For this review, take the finished solid that the model builds, in its own axes (mm). Face numbers are marked on the shaded views. Coordinates: 2 decimals unless noted, no trailing zeros. Loops run counter-clockwise (first coordinate to the right, second up) from the corner with the lowest first, then second, coordinate; pieces in that order, holes last.
1. Mouldability with a two-part tool opening along Z and no side actions: class the marked faces 1, 2 and 3 as pulls with the +Z half, pulls with the -Z half, needs draft (parallel to the pull), parting line crosses it, or undercut.
2. To check wall thickness, follow probe 1 along X at (y, z) = (-49, 77); probe 2 along X at (y, z) = (-4, 178); probe 3 along Y at (x, z) = (255, -86.5). State the ranges of each line that lie inside material, in increasing order.
3. Take a section at B-B, the plane y = -56.5. Count the separate pieces of the cut face and the enclosed holes in it, then the cut area to 3 significant figures.
4. Take a section at A-A, the plane z = 0. State the section outline as (x, y) points.
5. Clearance check with flat-ended pins moving along their axes: P1, Ø8, axis at x = 38.5, y = -46.5, coming from the -Z side (3 decimals); P2, Ø13, axis at x = -284.5, y = -89.5, coming from the +Z side; P3, Ø13.5, axis at x = -197.28, z = -197.28, coming from the +Y side; P4, Ø2, axis at y = -46, z = -125.5, coming from the +X side. State where each tip first meets the part, or that it passes through.
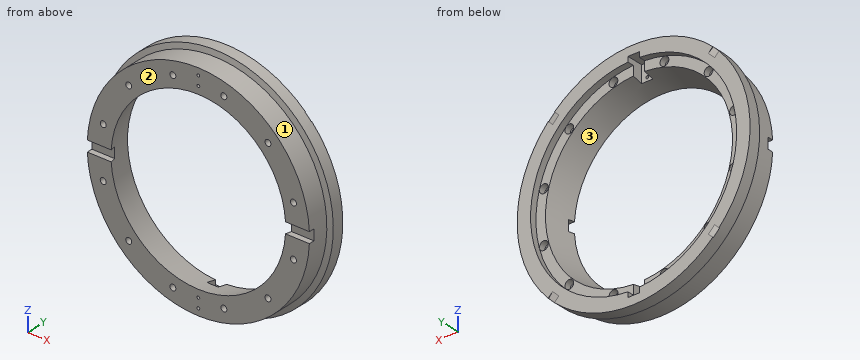
```python
from build123d import *

# Parameters (mm, degrees)
CUT_EXTRUDE_1_REACH = 475.247
SKETCH_2_R          = 8.5
SKETCH_3_R          = 12.5
CUT_EXTRUDE_2_DEPTH = 18
SKETCH_4_W          = 32
SKETCH_4_H          = 49.5
CUT_EXTRUDE_3_DEPTH = 47.5
CUT_EXTRUDE_4_REACH = 471.308
SKETCH_7_R          = 4
SKETCH_8_W          = 131
SKETCH_8_H          = 30.5
CUT_EXTRUDE_5_DEPTH = 16
CUT_REVOLVE_1_ANGLE = 5
CUT_REVOLVE_3_ANGLE = 5
CUT_REVOLVE_4_ANGLE = 5
CUT_REVOLVE_5_ANGLE = 5


with BuildPart() as part:
    # Sketch 1 → Revolve 1 (revolve)
    with BuildSketch(Plane.XY, mode=Mode.PRIVATE) as revolve_1_sk:
        Polygon((-330, 0), (-292, 0), (-292, -18.5), (-265, -18.5), (-247.5, -97), (-315, -97), (-315, -37.02), (-330, -33), align=None)
    revolve(revolve_1_sk.sketch.rotate(Axis((0, 0, 0), (0, 1, 0)), 270), axis=Axis((0, 0, 0), (0, 1, 0)))

    # Sketch 2 → Cut-Extrude 1 (cut, up to next)
    with BuildSketch(Plane(origin=(0, -18.5, 0), x_dir=(1, 0, 0), z_dir=(0, 1, 0)), mode=Mode.PRIVATE) as cut_extrude_1_sk1:
        with Locations(Location((-72.210513584, 269.493305535, 0), (0, 0, 270))):
            Circle(SKETCH_2_R)
    cut_extrude_1_tool1 = extrude(cut_extrude_1_sk1.sketch, amount=-CUT_EXTRUDE_1_REACH, mode=Mode.PRIVATE) & part.part
    # Sketch 2 → Cut-Extrude 1 (cut, up to next)
    with BuildSketch(Plane(origin=(0, -18.5, 0), x_dir=(1, 0, 0), z_dir=(0, 1, 0)), mode=Mode.PRIVATE) as cut_extrude_1_sk2:
        with Locations(Location((72.210513584, 269.493305535, 0), (0, 0, 270))):
            Circle(SKETCH_2_R)
    cut_extrude_1_tool2 = extrude(cut_extrude_1_sk2.sketch, amount=-CUT_EXTRUDE_1_REACH, mode=Mode.PRIVATE) & part.part
    # Sketch 2 → Cut-Extrude 1 (cut, up to next)
    with BuildSketch(Plane(origin=(0, -18.5, 0), x_dir=(1, 0, 0), z_dir=(0, 1, 0)), mode=Mode.PRIVATE) as cut_extrude_1_sk3:
        with Locations(Location((197.282791951, 197.282791951, 0), (0, 0, 270))):
            Circle(SKETCH_2_R)
    cut_extrude_1_tool3 = extrude(cut_extrude_1_sk3.sketch, amount=-CUT_EXTRUDE_1_REACH, mode=Mode.PRIVATE) & part.part
    # Sketch 2 → Cut-Extrude 1 (cut, up to next)
    with BuildSketch(Plane(origin=(0, -18.5, 0), x_dir=(1, 0, 0), z_dir=(0, 1, 0)), mode=Mode.PRIVATE) as cut_extrude_1_sk4:
        with Locations(Location((269.493305535, 72.210513584, 0), (0, 0, 270))):
            Circle(SKETCH_2_R)
    cut_extrude_1_tool4 = extrude(cut_extrude_1_sk4.sketch, amount=-CUT_EXTRUDE_1_REACH, mode=Mode.PRIVATE) & part.part
    # Sketch 2 → Cut-Extrude 1 (cut, up to next)
    with BuildSketch(Plane(origin=(0, -18.5, 0), x_dir=(1, 0, 0), z_dir=(0, 1, 0)), mode=Mode.PRIVATE) as cut_extrude_1_sk5:
        with Locations(Location((269.493305535, -72.210513584, 0), (0, 0, 270))):
            Circle(SKETCH_2_R)
    cut_extrude_1_tool5 = extrude(cut_extrude_1_sk5.sketch, amount=-CUT_EXTRUDE_1_REACH, mode=Mode.PRIVATE) & part.part
    # Sketch 2 → Cut-Extrude 1 (cut, up to next)
    with BuildSketch(Plane(origin=(0, -18.5, 0), x_dir=(1, 0, 0), z_dir=(0, 1, 0)), mode=Mode.PRIVATE) as cut_extrude_1_sk6:
        with Locations(Location((197.282791951, -197.282791951, 0), (0, 0, 270))):
            Circle(SKETCH_2_R)
    cut_extrude_1_tool6 = extrude(cut_extrude_1_sk6.sketch, amount=-CUT_EXTRUDE_1_REACH, mode=Mode.PRIVATE) & part.part
    # Sketch 2 → Cut-Extrude 1 (cut, up to next)
    with BuildSketch(Plane(origin=(0, -18.5, 0), x_dir=(1, 0, 0), z_dir=(0, 1, 0)), mode=Mode.PRIVATE) as cut_extrude_1_sk7:
        with Locations(Location((72.210513584, -269.493305535, 0), (0, 0, 270))):
            Circle(SKETCH_2_R)
    cut_extrude_1_tool7 = extrude(cut_extrude_1_sk7.sketch, amount=-CUT_EXTRUDE_1_REACH, mode=Mode.PRIVATE) & part.part
    # Sketch 2 → Cut-Extrude 1 (cut, up to next)
    with BuildSketch(Plane(origin=(0, -18.5, 0), x_dir=(1, 0, 0), z_dir=(0, 1, 0)), mode=Mode.PRIVATE) as cut_extrude_1_sk8:
        with Locations(Location((-72.210513584, -269.493305535, 0), (0, 0, 270))):
            Circle(SKETCH_2_R)
    cut_extrude_1_tool8 = extrude(cut_extrude_1_sk8.sketch, amount=-CUT_EXTRUDE_1_REACH, mode=Mode.PRIVATE) & part.part
    # Sketch 2 → Cut-Extrude 1 (cut, up to next)
    with BuildSketch(Plane(origin=(0, -18.5, 0), x_dir=(1, 0, 0), z_dir=(0, 1, 0)), mode=Mode.PRIVATE) as cut_extrude_1_sk9:
        with Locations(Location((-197.282791951, -197.282791951, 0), (0, 0, 270))):
            Circle(SKETCH_2_R)
    cut_extrude_1_tool9 = extrude(cut_extrude_1_sk9.sketch, amount=-CUT_EXTRUDE_1_REACH, mode=Mode.PRIVATE) & part.part
    # Sketch 2 → Cut-Extrude 1 (cut, up to next)
    with BuildSketch(Plane(origin=(0, -18.5, 0), x_dir=(1, 0, 0), z_dir=(0, 1, 0)), mode=Mode.PRIVATE) as cut_extrude_1_sk10:
        with Locations(Location((-269.493305535, -72.210513584, 0), (0, 0, 270))):
            Circle(SKETCH_2_R)
    cut_extrude_1_tool10 = extrude(cut_extrude_1_sk10.sketch, amount=-CUT_EXTRUDE_1_REACH, mode=Mode.PRIVATE) & part.part
    # Sketch 2 → Cut-Extrude 1 (cut, up to next)
    with BuildSketch(Plane(origin=(0, -18.5, 0), x_dir=(1, 0, 0), z_dir=(0, 1, 0)), mode=Mode.PRIVATE) as cut_extrude_1_sk11:
        with Locations(Location((-269.493305535, 72.210513584, 0), (0, 0, 270))):
            Circle(SKETCH_2_R)
    cut_extrude_1_tool11 = extrude(cut_extrude_1_sk11.sketch, amount=-CUT_EXTRUDE_1_REACH, mode=Mode.PRIVATE) & part.part
    # Sketch 2 → Cut-Extrude 1 (cut, up to next)
    with BuildSketch(Plane(origin=(0, -18.5, 0), x_dir=(1, 0, 0), z_dir=(0, 1, 0)), mode=Mode.PRIVATE) as cut_extrude_1_sk12:
        with Locations(Location((-197.282791951, 197.282791951, 0), (0, 0, 270))):
            Circle(SKETCH_2_R)
    cut_extrude_1_tool12 = extrude(cut_extrude_1_sk12.sketch, amount=-CUT_EXTRUDE_1_REACH, mode=Mode.PRIVATE) & part.part
    add(cut_extrude_1_tool1.solids().sort_by_distance((-72.210514, -18.5, -269.493306))[0], mode=Mode.SUBTRACT)
    add(cut_extrude_1_tool2.solids().sort_by_distance((72.210514, -18.5, -269.493306))[0], mode=Mode.SUBTRACT)
    add(cut_extrude_1_tool3.solids().sort_by_distance((197.282792, -18.5, -197.282792))[0], mode=Mode.SUBTRACT)
    add(cut_extrude_1_tool4.solids().sort_by_distance((269.493306, -18.5, -72.210514))[0], mode=Mode.SUBTRACT)
    add(cut_extrude_1_tool5.solids().sort_by_distance((269.493306, -18.5, 72.210514))[0], mode=Mode.SUBTRACT)
    add(cut_extrude_1_tool6.solids().sort_by_distance((197.282792, -18.5, 197.282792))[0], mode=Mode.SUBTRACT)
    add(cut_extrude_1_tool7.solids().sort_by_distance((72.210514, -18.5, 269.493306))[0], mode=Mode.SUBTRACT)
    add(cut_extrude_1_tool8.solids().sort_by_distance((-72.210514, -18.5, 269.493306))[0], mode=Mode.SUBTRACT)
    add(cut_extrude_1_tool9.solids().sort_by_distance((-197.282792, -18.5, 197.282792))[0], mode=Mode.SUBTRACT)
    add(cut_extrude_1_tool10.solids().sort_by_distance((-269.493306, -18.5, 72.210514))[0], mode=Mode.SUBTRACT)
    add(cut_extrude_1_tool11.solids().sort_by_distance((-269.493306, -18.5, -72.210514))[0], mode=Mode.SUBTRACT)
    add(cut_extrude_1_tool12.solids().sort_by_distance((-197.282792, -18.5, -197.282792))[0], mode=Mode.SUBTRACT)

    # Sketch 3 → Cut-Extrude 2 (cut)
    with BuildSketch(Plane(origin=(0, -18.5, 0), x_dir=(1, 0, 0), z_dir=(0, 1, 0))):
        with Locations(Location((-72.210513584, 269.493305535, 0), (0, 0, 270))):
            Circle(SKETCH_3_R)
        with Locations(Location((72.210513584, 269.493305535, 0), (0, 0, 270))):
            Circle(SKETCH_3_R)
        with Locations(Location((197.282791951, 197.282791951, 0), (0, 0, 270))):
            Circle(SKETCH_3_R)
        with Locations(Location((269.493305535, 72.210513584, 0), (0, 0, 270))):
            Circle(SKETCH_3_R)
        with Locations(Location((269.493305535, -72.210513584, 0), (0, 0, 270))):
            Circle(SKETCH_3_R)
        with Locations(Location((197.282791951, -197.282791951, 0), (0, 0, 270))):
            Circle(SKETCH_3_R)
        with Locations(Location((72.210513584, -269.493305535, 0), (0, 0, 270))):
            Circle(SKETCH_3_R)
        with Locations(Location((-72.210513584, -269.493305535, 0), (0, 0, 270))):
            Circle(SKETCH_3_R)
        with Locations(Location((-197.282791951, -197.282791951, 0), (0, 0, 270))):
            Circle(SKETCH_3_R)
        with Locations(Location((-269.493305535, -72.210513584, 0), (0, 0, 270))):
            Circle(SKETCH_3_R)
        with Locations(Location((-269.493305535, 72.210513584, 0), (0, 0, 270))):
            Circle(SKETCH_3_R)
        with Locations(Location((-197.282791951, 197.282791951, 0), (0, 0, 270))):
            Circle(SKETCH_3_R)
    extrude(amount=-CUT_EXTRUDE_2_DEPTH, mode=Mode.SUBTRACT)

    # Sketch 4 → Cut-Extrude 3 (cut)
    with BuildSketch(Plane(origin=(0, 0, 0), x_dir=(1, 0, 0), z_dir=(0, 1, 0))):
        with Locations((0, 281.25)):
            Rectangle(SKETCH_4_W, SKETCH_4_H)
        with Locations((0, -281.25)):
            Rectangle(SKETCH_4_W, SKETCH_4_H)
    extrude(amount=-CUT_EXTRUDE_3_DEPTH, mode=Mode.SUBTRACT)

    # Sketch 7 → Cut-Extrude 4 (cut, up to next)
    with BuildSketch(Plane(origin=(0, -47.5, 0), x_dir=(1, 0, 0), z_dir=(0, 1, 0)), mode=Mode.PRIVATE) as cut_extrude_4_sk1:
        with Locations(Location((0, 295.519729782, 0), (0, 0, 270))):
            Circle(SKETCH_7_R)
    cut_extrude_4_tool1 = extrude(cut_extrude_4_sk1.sketch, amount=-CUT_EXTRUDE_4_REACH, mode=Mode.PRIVATE) & part.part
    # Sketch 7 → Cut-Extrude 4 (cut, up to next)
    with BuildSketch(Plane(origin=(0, -47.5, 0), x_dir=(1, 0, 0), z_dir=(0, 1, 0)), mode=Mode.PRIVATE) as cut_extrude_4_sk2:
        with Locations(Location((0, 268.519729782, 0), (0, 0, 270))):
            Circle(SKETCH_7_R)
    cut_extrude_4_tool2 = extrude(cut_extrude_4_sk2.sketch, amount=-CUT_EXTRUDE_4_REACH, mode=Mode.PRIVATE) & part.part
    # Sketch 7 → Cut-Extrude 4 (cut, up to next)
    with BuildSketch(Plane(origin=(0, -47.5, 0), x_dir=(1, 0, 0), z_dir=(0, 1, 0)), mode=Mode.PRIVATE) as cut_extrude_4_sk3:
        with Locations(Location((0, -268.519729782, 0), (0, 0, 270))):
            Circle(SKETCH_7_R)
    cut_extrude_4_tool3 = extrude(cut_extrude_4_sk3.sketch, amount=-CUT_EXTRUDE_4_REACH, mode=Mode.PRIVATE) & part.part
    # Sketch 7 → Cut-Extrude 4 (cut, up to next)
    with BuildSketch(Plane(origin=(0, -47.5, 0), x_dir=(1, 0, 0), z_dir=(0, 1, 0)), mode=Mode.PRIVATE) as cut_extrude_4_sk4:
        with Locations(Location((0, -295.519729782, 0), (0, 0, 270))):
            Circle(SKETCH_7_R)
    cut_extrude_4_tool4 = extrude(cut_extrude_4_sk4.sketch, amount=-CUT_EXTRUDE_4_REACH, mode=Mode.PRIVATE) & part.part
    add(cut_extrude_4_tool1.solids().sort_by_distance((0, -47.5, -295.51973))[0], mode=Mode.SUBTRACT)
    add(cut_extrude_4_tool2.solids().sort_by_distance((0, -47.5, -268.51973))[0], mode=Mode.SUBTRACT)
    add(cut_extrude_4_tool3.solids().sort_by_distance((0, -47.5, 268.51973))[0], mode=Mode.SUBTRACT)
    add(cut_extrude_4_tool4.solids().sort_by_distance((0, -47.5, 295.51973))[0], mode=Mode.SUBTRACT)

    # Sketch 8 → Cut-Extrude 5 (cut)
    with BuildSketch(Plane.XZ.offset(97)):
        with Locations((285.5, 0)):
            Rectangle(SKETCH_8_W, SKETCH_8_H)
        with Locations((-285.5, 0)):
            Rectangle(SKETCH_8_W, SKETCH_8_H)
    extrude(amount=-CUT_EXTRUDE_5_DEPTH, mode=Mode.SUBTRACT)

    # Sketch 9 → Cut-Revolve 1 (revolve, cut)
    with BuildSketch(Plane(origin=(0, 0, 0), x_dir=(1, 0, 0), z_dir=(0, 1, 0))):
        Polygon((-237.834010658, 255.511680188), (-255.511680188, 237.834010658), (-229.563996686, 211.886327157), (-211.886327157, 229.563996686), align=None)
    revolve(axis=Axis((-211.886327157, 0, -229.563996686), (-0.7071067811865481, 0, 0.707106781186547)), revolution_arc=CUT_REVOLVE_1_ANGLE, mode=Mode.SUBTRACT)

    # Sketch 9_3 → Cut-Revolve 3 (revolve, cut)
    with BuildSketch(Plane(origin=(0, 0, 0), x_dir=(1, 0, 0), z_dir=(0, 1, 0))):
        Polygon((255.511680188, 237.834010658), (237.834010658, 255.511680188), (211.886327157, 229.563996686), (229.563996686, 211.886327157), align=None)
    revolve(axis=Axis((229.563996686, 0, -211.886327157), (-0.7071067811865481, 0, -0.707106781186547)), revolution_arc=CUT_REVOLVE_3_ANGLE, mode=Mode.SUBTRACT)

    # Sketch 9_4 → Cut-Revolve 4 (revolve, cut)
    with BuildSketch(Plane(origin=(0, 0, 0), x_dir=(1, 0, 0), z_dir=(0, 1, 0))):
        Polygon((237.834010658, -255.511680188), (255.511680188, -237.834010658), (229.563996686, -211.886327156), (211.886327157, -229.563996686), align=None)
    revolve(axis=Axis((211.886327157, 0, 229.563996686), (0.7071067811865481, 0, -0.707106781186547)), revolution_arc=CUT_REVOLVE_4_ANGLE, mode=Mode.SUBTRACT)

    # Sketch 9_5 → Cut-Revolve 5 (revolve, cut)
    with BuildSketch(Plane(origin=(0, 0, 0), x_dir=(1, 0, 0), z_dir=(0, 1, 0))):
        Polygon((-255.511680188, -237.834010658), (-237.834010658, -255.511680188), (-211.886327156, -229.563996686), (-229.563996686, -211.886327157), align=None)
    revolve(axis=Axis((-229.563996686, 0, 211.886327157), (0.7071067811865481, 0, 0.707106781186547)), revolution_arc=CUT_REVOLVE_5_ANGLE, mode=Mode.SUBTRACT)


solid = part.part
```
Results list:
1. face 1: parting line crosses it
1. face 2: needs draft
1. face 3: undercut
2. probe 1: x = -305.44 to -276.52, -262.47 to -246.45, 246.45 to 262.47, 276.52 to 305.44
2. probe 2: x = -277.88 to -231.47, 231.47 to 277.88
2. probe 3: y = -97 to -18.5
3. separate pieces: 1
3. enclosed holes: 17
3. area: 102,000 mm2
4. outline: (-330, -33) - (-315, -37.02) - (-315, -81) - (-251.07, -81) - (-265, -18.5) - (-292, -18.5) - (-292, 0) - (-330, 0) - close; (251.07, -81) - (315, -81) - (315, -37.02) - (330, -33) - (330, 0) - (292, 0) - (292, -18.5) - (265, -18.5) - close
5. P1: stops at z = -313.105
5. P2: stops at z = 148.12
5. P3: passes through
5. P4: stops at x = 289.35
